Answer from the drawing. Dimensions are ordinates in mm from the lowest x, y and z of the part. A direction names the side the tool comes from. Round coordinates to 2 decimals unless told otherwise and drop trailing zeros. Loops run counter-clockwise (first coordinate to the right, second up) from the corner with the lowest first, then second, coordinate; pieces in that order, holes last. Notation, with made-up numbers: M 58,33 L 77,33 A30 ccw 77,63 Z; hole C 22.5,-23 d4. An arc over 180 degrees is marked long. One line per item, written item: value.
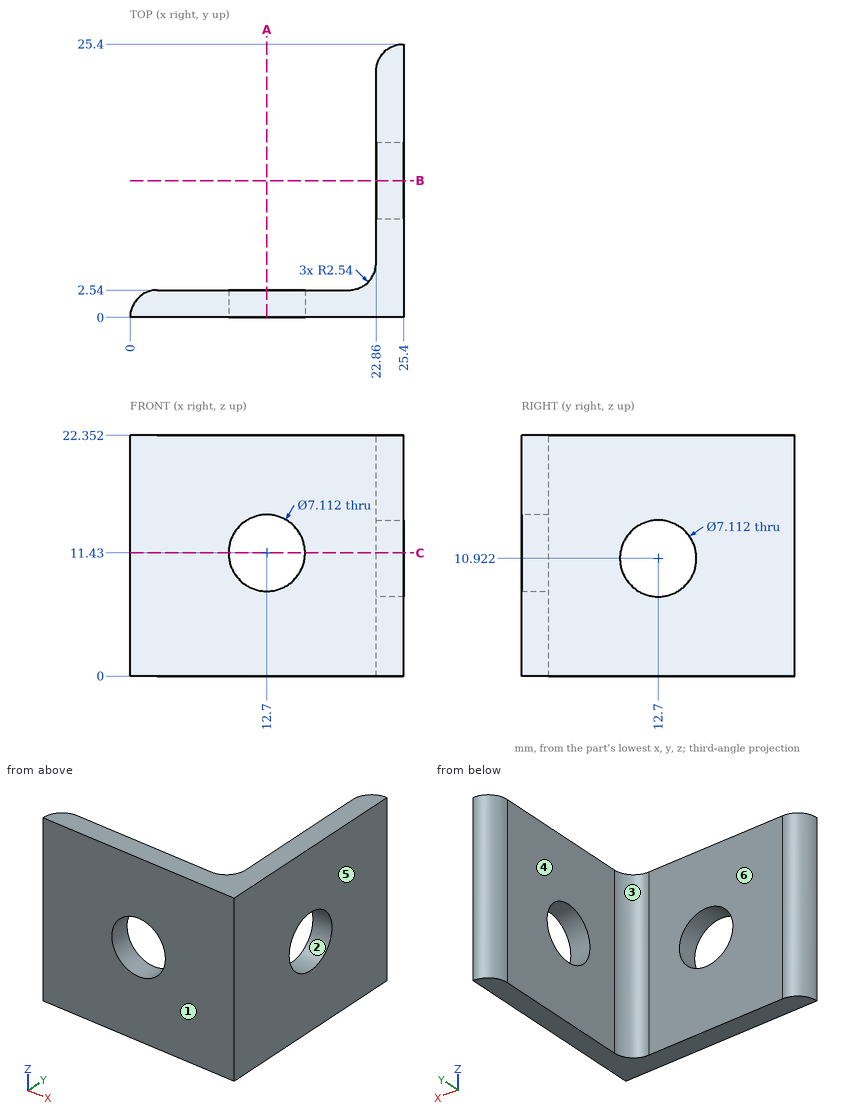
1) For the marked faces 5 and 6, determine the directions among +Z, -Z, +X, -X, +Y, -Y from which every point of the face is accessible in a straight line to the end or side of a thin tool.
Check values:
face 5: +Z, -Z, +X, +Y, -Y
face 6: +Z, -Z, -X, +Y
2) Each of these flat-tipped pins is pushed along its axis until it touches: pin 1 (5 mm diameter, centred on y = 11, z = 11.5, fed in from -X); pin 2 (1.5 mm diameter, centred on x = 18.5, z = 20, fed in from -Y). Where does it stop, or does it pass through?
Check values:
pin 1: x = 22.86
pin 2: y = 0
3) Find the intervals of material crossed by probe 1 along X at (y, z) = (21.75, 19.25); probe 2 along Y at (x, z) = (19.75, 8); probe 3 along X at (y, z) = (0.95, 11.43), in increasing order. Write a range as from..to.
Check values:
probe 1: 22.86..25.4
probe 2: 0..2.54
probe 3: 0.18..9.14, 16.26..25.4
4) The mould has two halves that part along Y. Classify the marked faces 1, 2, 3 and 4: +Y half, -Y half, draft (parallel to the pull), parting line (faces both ways), or undercut.
Check values:
face 1: -Y half
face 2: undercut
face 3: +Y half
face 4: draft
5) Find section A-A (x = 12.7). Give the vertices of the cut face in (y, z).
Check values:
outline: M 0,0 L 2.54,0 L 2.54,7.87 L 0,7.87 Z; M 0,14.99 L 2.54,14.99 L 2.54,22.35 L 0,22.35 Z
6) Find section C-C (z = 11.43). Give the number of separate pieces and of enclosed holes in the cut face.
Check values:
separate pieces: 3
enclosed holes: 0
7) Find section B-B (y = 12.7). Give the vertices of the cut face in (x, z).
Check values:
outline: M 22.86,0 L 25.4,0 L 25.4,7.37 L 22.86,7.37 Z; M 22.86,14.48 L 25.4,14.48 L 25.4,22.35 L 22.86,22.35 Z
